Read the model definition and answer for the solid it produces. Units are mm, in the model's axes. Face numbers are marked on the shaded views. A direction names the side the tool comes from. Give positions to 0.01 mm unless a question says otherwise; leave off trailing zeros. Loops run counter-clockwise (first coordinate to the right, second up) from the corner with the lowest first, then second, coordinate; pieces in that order, holes last. Notation, with made-up numbers: M 59,51.5 L 71,51.5 A13 cw 71,67.5 Z; hole C -18.5,1.5 d10. An arc over 180 degrees is marked long. Return JSON: item names as keys, results as strings. Group by question number.
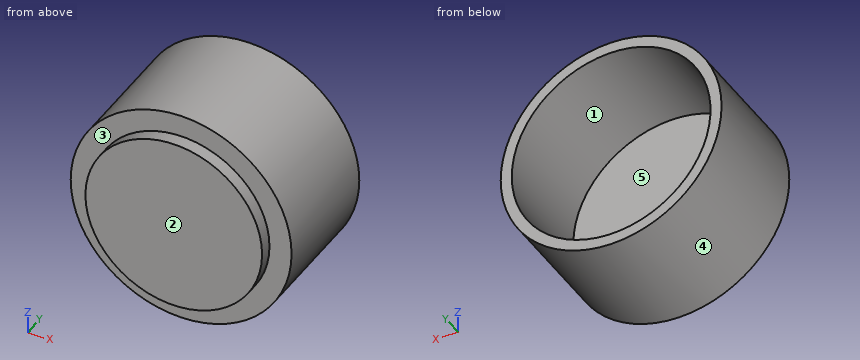
Autodesk Inventor part; units mm, degrees
ref_plane "YZ Plane" through (0, 0, 0) normal (1, 0, 0) x (0, 1, 0)
ref_plane "XZ Plane" through (0, 0, 0) normal (0, 1, 0) x (-1, 0, 0)
ref_plane "XY Plane" through (0, 0, 0) normal (0, 0, 1) x (1, 0, 0)
sketch "Boceto1" plane through (0, 0, 0) normal (0, 1, 0) x (-1, 0, 0)
  circle A0 centre (0, 0) radius 50
  dimension "d0" = 100
extrude "Extrusión1" add sketch "Boceto1" along normal blind 55
sketch "Boceto2" plane through (0, 55, 0) normal (0, 1, 0) x (1, 0, 0)
  circle A0 centre (0, 0) radius 45
  dimension "d3" = 90
extrude "Extrusión2" cut sketch "Boceto2" against normal blind 50
thread "Rosca1"
sketch "Boceto3" plane through (0, 0, 0) normal (0, -1, 0) x (1, 0, 0)
  circle A0 centre (0, 0) radius 40
  dimension "d8" = 80
extrude "Extrusión3" add sketch "Boceto3" along normal blind 6
thread "Rosca2"
1. Find section B-B (y = 39). Write down the section's boundary in (x, z), and give its area (3 significant figures).
2. For the marked faces 1 and 2, determine the directions among +Z, -Z, +X, -X, +Y, -Y from which every point of the face is accessible in a straight line to the end or side of a thin tool.
3. Flat-ended cylindrical pins translate along their axes: P1, Ø8, axis at x = -34, y = 9, coming from the -Z side; P2, Ø12, axis at x = 32.5, y = 17, coming from the +Z side; P3, Ø5, axis at x = -1, z = 21, coming from the +Y side. Find the tip coordinate at first contact, or state that the pin passes through.
4. Find section D-D (z = 43.5). Write down the section's boundary in (x, y), and give its area (3 significant figures).
5. Find section C-C (x = 0). Write down the section's boundary in (y, z).
6. Find section A-A (z = 0). Write down the section's boundary in (x, y), and give its area (3 significant figures).
7. Straight lines are drawn through the part: line 1 along Z through (x, y) = (0, 29); line 2 along Y through (x, z) = (21, 25.5); line 3 along Y through (x, z) = (19.5, 37). For each, find the intervals that lie inside material, in ascending order.
8. The mould has two halves that part along X. Classify the marked faces 3, 4 and 5: +X half, -X half, draft (parallel to the pull), parting line (faces both ways), or undercut.
Result:
{
 "1": {"outline": "C 0,0 d100; hole C 0,0 d90", "area": "1,490 mm2"},
 "2": {"face 1": "+Y", "face 2": "+Z, -Z, +X, -X, -Y"},
 "3": {"P1": "stops at z = -40", "P2": "stops at z = 42.4", "P3": "stops at y = 5"},
 "4": {"outline": "M -24.65,0 L 24.65,0 L 24.65,55 L 11.52,55 L 11.52,5 L -11.52,5 L -11.52,55 L -24.65,55 Z", "area": "1,560 mm2"},
 "5": {"outline": "M -6,-40 L 0,-40 L 0,-50 L 55,-50 L 55,-45 L 5,-45 L 5,45 L 55,45 L 55,50 L 0,50 L 0,40 L -6,40 Z"},
 "6": {"outline": "M -50,0 L -40,0 L -40,-6 L 40,-6 L 40,0 L 50,0 L 50,55 L 45,55 L 45,5 L -45,5 L -45,55 L -50,55 Z", "area": "1,480 mm2"},
 "7": {"line 1": "z = -50 to -45, 45 to 50", "line 2": "y = -6 to 5", "line 3": "y = 0 to 5"},
 "8": {"face 3": "draft", "face 4": "parting line", "face 5": "undercut"}
}
